Could you check a few things on this model? Use its own coordinates, in mm. A direction names the side the tool comes from. Coordinates: 2 decimals unless noted, no trailing zeros. Loops run counter-clockwise (first coordinate to the right, second up) from the corner with the lowest first, then second, coordinate; pieces in that order, holes last.
1) Imagine slicing it at A-A on y = 2.05. Please give me the cut outline in (x, z).
2) Thinking about a two-plate mould opening in X: for faces 5 (the face through (1.5, 1.5, 11)), 6 (the face through (-4.057, 1.458, 11.121)), 7 (the face through (-2, 1, 13.5)), which applies, released by +X, released by -X, zero draft, split by the parting line, or undercut?
3) For faces 1 (the face through (4, 2, 3.1)), 2 (the face through (-1.5, 1.5, 11)), 3 (the face through (0.85, -1, 6)), 4 (the face through (-1.708, 2.218, 6.479)), which set-ups out of +Z, -Z, +X, -X, +Y, -Y let a thin tool reach every point of the face, with its end or its side?
4) Imagine slicing it at B-B on z = 4.25. Please give me the cut outline in (x, y), plus the area to 3 significant figures.
5) If I drill on line 1 along X through (y, z) = (-1, 0); line 2 along Z through (x, y) = (0, -0.9); line 3 along X through (y, z) = (0.85, 4), over which ranges is the centre line in solid material (lowest first)?
6) Will these pins go through, and if not, where does the flat tip stop? P1, Ø2, axis at x = 1, z = 11.5, coming from the -Y side; P2, Ø1.5, axis at x = -3.5, y = 3.5, coming from the -Z side.
7) Imagine slicing it at C-C on x = -2. Please give me the cut outline in (y, z), plus the area to 3 significant figures.
8) Imagine slicing it at D-D on y = -0.2. Please give me the cut outline in (x, z), plus the area to 3 significant figures.
```python
from build123d import *

# Parameters (mm, degrees)
F1_DEPTH = 1.5
F3_DEPTH = 4.5
F4_R     = 0.5


with BuildPart() as f1:
    # F0 (on Front) → F1 (new body)
    with BuildSketch(Plane.XZ):
        with BuildLine():
            ThreePointArc((0.85, 2.9811910372), (0, -3.1), (-0.85, 2.9811910372))
            Line((-0.85, 2.9811910372), (-0.85, 9.7640792906))
            ThreePointArc((-0.85, 9.7640792906), (-1.5, 11), (-0.85, 12.2359207094))
            Line((-0.85, 12.2359207094), (-0.85, 13.5))
            Line((-0.85, 13.5), (-3, 13.5))
            Line((-3, 13.5), (-5, 9))
            Line((-5, 9), (-5, 0))
            ThreePointArc((-5, 0), (0, -5), (5, 0))
            Line((5, 0), (5, 9))
            Line((5, 9), (3, 13.5))
            Line((3, 13.5), (0.85, 13.5))
            Line((0.85, 13.5), (0.85, 12.2359207094))
            ThreePointArc((0.85, 12.2359207094), (1.5, 11), (0.85, 9.7640792906))
            Line((0.85, 9.7640792906), (0.85, 2.9811910372))
        make_face()
    extrude(amount=F1_DEPTH)

    # F2 (on face) → F3 (join)
    with BuildSketch(Plane(origin=(0, 0, 0), x_dir=(-1, 0, 0), z_dir=(0, 1, 0))):
        with BuildLine():
            Line((0.85, 9.7640792906), (2.590399856, 3.1))
            Line((2.590399856, 3.1), (5, 3.1))
            Line((5, 3.1), (5, 9))
            Line((5, 9), (3, 13.5))
            Line((3, 13.5), (0.85, 13.5))
            Line((0.85, 13.5), (0.85, 12.2359207094))
            ThreePointArc((0.85, 12.2359207094), (1.5, 11), (0.85, 9.7640792906))
        make_face()
        with BuildLine():
            Line((-5, 3.1), (-2.590399856, 3.1))
            Line((-2.590399856, 3.1), (-0.85, 9.7640792906))
            ThreePointArc((-0.85, 9.7640792906), (-1.5, 11), (-0.85, 12.2359207094))
            Line((-0.85, 12.2359207094), (-0.85, 13.5))
            Line((-0.85, 13.5), (-3, 13.5))
            Line((-3, 13.5), (-5, 9))
            Line((-5, 9), (-5, 3.1))
        make_face()
    extrude(amount=F3_DEPTH)

    # F4
    f4_edges = [f1.edges().sort_by_distance(p)[0] for p in [
        (3, 1.5, 13.5),
        (5, 1.5, 9),
        (-3, 1.5, 13.5),
        (-5, 1.5, 9),
        (0.85, 1.5, 13.5),
        (-0.85, 1.5, 13.5),
        (5, 2.25, 3.1),
        (-5, 2.25, 3.1),
    ]]
    fillet(f4_edges, radius=F4_R)


solid = f1.part
```
Filled in:
1. outline: (-5, 3.6) arc R0.5 ccw to (-4.5, 3.1) - (-2.59, 3.1) - (-0.85, 9.76) arc R1.5 cw to (-0.85, 12.24) - (-0.85, 13) arc R0.5 ccw to (-1.35, 13.5) - (-2.68, 13.5) arc R0.5 ccw to (-3.13, 13.2) - (-4.96, 9.1) arc R0.5 ccw to (-5, 8.89) - close; (0.85, 9.76) - (2.59, 3.1) - (4.5, 3.1) arc R0.5 ccw to (5, 3.6) - (5, 8.89) arc R0.5 ccw to (4.96, 9.1) - (3.13, 13.2) arc R0.5 ccw to (2.68, 13.5) - (1.35, 13.5) arc R0.5 ccw to (0.85, 13) - (0.85, 12.24) arc R1.5 cw to start
2. face 5: undercut
2. face 6: released by -X
2. face 7: zero draft
3. face 1: -Z, +X, -X, +Y
3. face 2: +Y, -Y
3. face 3: +Z, +Y, -Y
3. face 4: -Z, +Y
4. outline: (-5, -1.5) - (-0.85, -1.5) - (-0.85, 0) - (-2.29, 0) - (-2.29, 4.5) - (-5, 4.5) - close; (0.85, -1.5) - (5, -1.5) - (5, 4.5) - (2.29, 4.5) - (2.29, 0) - (0.85, 0) - close
4. area: 36.8 mm2
5. line 1: x = -5 to -3.1, 3.1 to 5
5. line 2: z = -5 to -3.1
5. line 3: x = -5 to -2.36, 2.36 to 5
6. P1: stops at y = -1.5
6. P2: stops at z = 3.1
7. outline: (-1.5, -4.58) - (0, -4.58) - (0, -2.37) - (-1.5, -2.37) - close; (-1.5, 2.37) - (0, 2.37) - (0, 5.36) - (4.5, 5.36) - (4.5, 13.5) - (-1.5, 13.5) - close
7. area: 56.6 mm2
8. outline: (-5, 0) arc R5 ccw to (5, 0) - (5, 8.89) arc R0.5 ccw to (4.96, 9.1) - (3.13, 13.2) arc R0.5 ccw to (2.68, 13.5) - (1.35, 13.5) arc R0.5 ccw to (0.85, 13) - (0.85, 12.24) arc R1.5 cw to (0.85, 9.76) - (0.85, 2.98) arc R3.1 cw (long way) to (-0.85, 2.98) - (-0.85, 9.76) arc R1.5 cw to (-0.85, 12.24) - (-0.85, 13) arc R0.5 ccw to (-1.35, 13.5) - (-2.68, 13.5) arc R0.5 ccw to (-3.13, 13.2) - (-4.96, 9.1) arc R0.5 ccw to (-5, 8.89) - close
8. area: 115 mm2
